Geometry check sheet. Reference: the model listing, model coordinates, mm. A direction names the side the tool comes from. Round coordinates to 2 decimals unless told otherwise and drop trailing zeros. Loops run counter-clockwise (first coordinate to the right, second up) from the corner with the lowest first, then second, coordinate; pieces in that order, holes last.
```python
from build123d import *

# Parameters (mm, degrees)
F0_W      = 2.999994
F0_H      = 110.000034
F0_H_2    = 36.83
F1_DEPTH  = 2.999994
F2_DEPTH  = 50.8
F3_DEPTH  = 36.999926
F4_R      = 2.1499957
F5_DEPTH  = 49.276
F6_R      = 5.969
F7_DEPTH  = 38.1
F8_R      = 2.54
F10_DEPTH = 5.08
F11_R     = 2.54
F12_DEPTH = 330.2
F13_R     = 2.54


with BuildPart() as f1:
    # F0 (on Top) → F1 (new body)
    with BuildSketch(Plane.XY):
        Rectangle(F0_W, F0_H)
        Polygon((38.085014, 18.415), (1.499997, 55.000017), (1.499997, -55.000017), (38.085014, -18.415), (201.500105, -18.415), (201.500105, 18.415), align=None)
        with Locations((203.000102, 0)):
            Rectangle(F0_W, F0_H_2)
    extrude(amount=F1_DEPTH)

    # F0 (on Top) → F2 (join)
    with BuildSketch(Plane.XY):
        Rectangle(F0_W, F0_H)
    extrude(amount=F2_DEPTH)

    # F0 (on Top) → F3 (join)
    with BuildSketch(Plane.XY):
        with Locations((203.000102, 0)):
            Rectangle(F0_W, F0_H_2)
    extrude(amount=F3_DEPTH)

    # F4 (on face) → F5 (cut)
    with BuildSketch(Plane.YZ.offset(1.499997)):
        with Locations((-44.840017, 43.18)):
            Circle(F4_R)
        with Locations((-44.840017, 13.18006)):
            Circle(F4_R)
        with Locations((-19.440017, 43.18)):
            Circle(F4_R)
        with Locations((-19.440017, 13.18006)):
            Circle(F4_R)
        with Locations((44.840017, 43.18)):
            Circle(F4_R)
        with Locations((19.440017, 43.18)):
            Circle(F4_R)
        with Locations((19.440017, 13.18006)):
            Circle(F4_R)
        with Locations((44.840017, 13.18006)):
            Circle(F4_R)
    extrude(amount=-F5_DEPTH, mode=Mode.SUBTRACT)

    # F6 (on face) → F7 (cut)
    with BuildSketch(Plane.YZ.offset(204.500099)):
        with Locations((0, 12.192)):
            Circle(F6_R)
    extrude(amount=-F7_DEPTH, mode=Mode.SUBTRACT)

    # F8
    f8_edges = [f1.edges().sort_by_distance(p)[0] for p in [
        (201.500105, 0, 2.999994),
    ]]
    fillet(f8_edges, radius=F8_R)

    # F9 (on face) → F10 (join)
    with BuildSketch(Plane.XY.offset(2.999994)):
        with BuildLine():
            ThreePointArc((92.4825774501, -18.415), (97.360105, -19.05), (102.2376325499, -18.415))
            Line((102.2376325499, -18.415), (92.4825774501, -18.415))
        make_face()
        with BuildLine():
            ThreePointArc((102.2376325499, -18.415), (112.4567834397, -11.6186401996), (116.410105, 0))
            ThreePointArc((116.410105, 0), (112.4567834397, 11.6186401996), (102.2376325499, 18.415))
            Line((102.2376325499, 18.415), (92.4825774501, 18.415))
            ThreePointArc((92.4825774501, 18.415), (78.310105, 0), (92.4825774501, -18.415))
            Line((92.4825774501, -18.415), (102.2376325499, -18.415))
        make_face()
        with BuildLine():
            Line((92.4825774501, 18.415), (102.2376325499, 18.415))
            ThreePointArc((102.2376325499, 18.415), (97.360105, 19.05), (92.4825774501, 18.415))
        make_face()
    extrude(amount=F10_DEPTH)

    # F11 (on face) → F12 (join)
    with BuildSketch(Plane.XY.offset(8.079994)):
        with Locations((97.360105, 0)):
            Circle(F11_R)
    extrude(amount=F12_DEPTH)

    # F13
    f13_edges = [f1.edges().sort_by_distance(p)[0] for p in [
        (1.499997, 0, 2.999994),
    ]]
    fillet(f13_edges, radius=F13_R)


solid = f1.part
```
1) Sectioned sample at C-C, the plane x = 150.5. Record the cut outline in (y, z) (3 decimals).
Report:
outline: (-18.415, 0) - (18.415, 0) - (18.415, 3) - (-18.415, 3) - close
2) Access from +Z, -Z, +X, -X, +Y, -Y to the whole of each face (thin tool, end or side, straight path). Record for faces 4 (the face through (201.5, 0, 21)), 5 (the face through (20, 36.5, 1.5)), 6 (the face through (203.021, -1.294, 6.365)).
Report:
face 4: +Z, +Y, -Y
face 5: +Z, -Z, +X, +Y
face 6: +X
3) Sectioned sample at B-B, the plane y = 31. Record the cut outline in (x, z), then the cut area to 3 significant figures.
Report:
outline: (-1.5, 0) - (25.5, 0) - (25.5, 3) - (4.04, 3) arc R2.54 cw to (1.5, 5.54) - (1.5, 50.8) - (-1.5, 50.8) - close
area: 226 mm2
4) Mould release check, pull along X, two halves, no side actions. Record for faces 1 (the face through (19.5, -37, 1.5)), 2 (the face through (101, 0, 8.08)), 3 (the face through (146, 18.415, 2)): +X half, -X half, draft (parallel to the pull), parting line (faces both ways), or undercut.
Report:
face 1: +X half
face 2: undercut
face 3: draft
5) Scan lines: line 1 along Z through (x, y) = (202, 0); line 2 along Z through (x, y) = (175, -4.5); line 3 along X through (y, z) = (-28.5, 16.5). Record each from-to range of solid material in increasing order.
Report:
line 1: z = 0 to 6.22, 18.16 to 37
line 2: z = 0 to 3
line 3: x = -1.5 to 1.5
6) Sectioned sample at A-A, the plane z = 285. Record the cut outline in (x, y).
Report:
outline: circle Ø5.08 at (97.36, 0)
7) Sectioned sample at D-D, the plane y = 10.5. Record the cut outline in (x, z).
Report:
outline: (-1.5, 0) - (204.5, 0) - (204.5, 37) - (201.5, 37) - (201.5, 5.54) arc R2.54 cw to (198.96, 3) - (113.26, 3) - (113.26, 8.08) - (81.47, 8.08) - (81.47, 3) - (4.04, 3) arc R2.54 cw to (1.5, 5.54) - (1.5, 50.8) - (-1.5, 50.8) - close
8) Gauge pin test, flat ends, axial feed: pin 1 (8 mm diameter, centred on x = 105, y = 3.5, fed in from +Z); pin 2 (10.5 mm diameter, centred on y = 0, z = 12.192, fed in from +X); pin 3 (4 mm diameter, centred on y = 44.84, z = 43.18, fed in from -X); pin 4 (8 mm diameter, centred on x = 97, z = 226, fed in from -Y). Record the tip position at first contact, or that the pin passes through.
Report:
pin 1: stops at z = 8.08
pin 2: stops at x = 116.41
pin 3: passes through
pin 4: stops at y = -2.54
